from build123d import *

# Parameters (mm, degrees)
SKETCH_1_W                         = 321
SKETCH_1_H                         = 60
SM_BASE_FLANGE_1_DEPTH             = 1.5
SM_EDGE_FLANGE_1_STRIP_W           = 6.2
SM_EDGE_FLANGE_1_STRIP_H           = 1.5
SM_EDGE_FLANGE_1_STRIP_CUT_DEPTH   = 321
SM_EDGE_FLANGE_1_STRIP_2_W         = 6.2
SM_EDGE_FLANGE_1_STRIP_2_H         = 1.5
SM_EDGE_FLANGE_1_STRIP_CUT_2_DEPTH = 321
SM_EDGE_FLANGE_1_DEPTH             = 321
SM_EDGE_FLANGE_1_BEND_DEPTH        = 321
SM_EDGE_FLANGE_2_STRIP_W           = 6.2
SM_EDGE_FLANGE_2_STRIP_H           = 1.5
SM_EDGE_FLANGE_2_STRIP_CUT_DEPTH   = 321
SM_EDGE_FLANGE_2_STRIP_2_W         = 6.2
SM_EDGE_FLANGE_2_STRIP_2_H         = 1.5
SM_EDGE_FLANGE_2_STRIP_CUT_2_DEPTH = 321
SM_EDGE_FLANGE_2_DEPTH             = 321
SM_EDGE_FLANGE_2_BEND_DEPTH        = 321
CUT_EXTRUDE_2_DEPTH                = 174.385408844
CUT_EXTRUDE_3_DEPTH                = 57
CUT_EXTRUDE_3_DEPTH_BACK           = 10
SKETCH_20_W                        = 341.087454661
SKETCH_20_H                        = 74.910603127
CUT_EXTRUDE_4_DEPTH                = 166.663061664
CUT_EXTRUDE_4_DEPTH_BACK           = 166.663061664
SKETCH_21_R                        = 0.75


# Sheet-metal steps are written as plain solids
with BuildPart() as part:
    # Sketch 1 → 基体-法兰1 (new body)
    with BuildSketch(Plane.XY):
        Rectangle(SKETCH_1_W, SKETCH_1_H)
    extrude(amount=-SM_BASE_FLANGE_1_DEPTH)

    # 边线-法兰1 strip (across the edge) → 边线-法兰1 strip cut (cut)
    with BuildSketch(Plane(origin=(160.5, 30, 0), x_dir=(0, -1, 0), z_dir=(-1, 0, 0))):
        with Locations((-1.5, -0.75)):
            Rectangle(SM_EDGE_FLANGE_1_STRIP_W, SM_EDGE_FLANGE_1_STRIP_H)
    extrude(amount=SM_EDGE_FLANGE_1_STRIP_CUT_DEPTH, mode=Mode.SUBTRACT)

    # 边线-法兰1 strip 2 (across the edge) → 边线-法兰1 strip cut 2 (cut)
    with BuildSketch(Plane(origin=(-160.5, -30, 0), x_dir=(0, 1, 0), z_dir=(1, 0, 0))):
        with Locations((-1.5, -0.75)):
            Rectangle(SM_EDGE_FLANGE_1_STRIP_2_W, SM_EDGE_FLANGE_1_STRIP_2_H)
    extrude(amount=SM_EDGE_FLANGE_1_STRIP_CUT_2_DEPTH, mode=Mode.SUBTRACT)

    # 边线-法兰1 section (across the edge) → 边线-法兰1 (add)
    with BuildSketch(Plane(origin=(160.5, 30, 0), x_dir=(0, -1, 0), z_dir=(-1, 0, 0))):
        with BuildLine():
            Line((0, 0.1), (0, 26.5))
            Line((0, 26.5), (1.5, 26.5))
            Line((1.5, 26.5), (1.5, 0.1))
            ThreePointArc((1.5, 0.1), (1.529289322, 0.029289322), (1.6, 0))
            Line((1.6, 0), (1.6, -1.5))
            ThreePointArc((1.6, -1.5), (0.46862915, -1.03137085), (0, 0.1))
        make_face()
    extrude(amount=SM_EDGE_FLANGE_1_DEPTH)

    # 边线-法兰1 section 2 (across the edge) → 边线-法兰1 bend (add)
    with BuildSketch(Plane(origin=(-160.5, -30, 0), x_dir=(0, 1, 0), z_dir=(1, 0, 0))):
        with BuildLine():
            Line((0, 0.1), (0, 26.5))
            Line((0, 26.5), (1.5, 26.5))
            Line((1.5, 26.5), (1.5, 0.1))
            ThreePointArc((1.5, 0.1), (1.529289322, 0.029289322), (1.6, 0))
            Line((1.6, 0), (1.6, -1.5))
            ThreePointArc((1.6, -1.5), (0.46862915, -1.03137085), (0, 0.1))
        make_face()
    extrude(amount=SM_EDGE_FLANGE_1_BEND_DEPTH)

    # 边线-法兰2 strip (across the edge) → 边线-法兰2 strip cut (cut)
    with BuildSketch(Plane(origin=(160.5, 28.5, 26.5), x_dir=(0, 0, -1), z_dir=(-1, 0, 0))):
        with Locations((-1.5, -0.75)):
            Rectangle(SM_EDGE_FLANGE_2_STRIP_W, SM_EDGE_FLANGE_2_STRIP_H)
    extrude(amount=SM_EDGE_FLANGE_2_STRIP_CUT_DEPTH, mode=Mode.SUBTRACT)

    # 边线-法兰2 strip 2 (across the edge) → 边线-法兰2 strip cut 2 (cut)
    with BuildSketch(Plane(origin=(-160.5, -28.5, 26.5), x_dir=(0, 0, -1), z_dir=(1, 0, 0))):
        with Locations((-1.5, -0.75)):
            Rectangle(SM_EDGE_FLANGE_2_STRIP_2_W, SM_EDGE_FLANGE_2_STRIP_2_H)
    extrude(amount=SM_EDGE_FLANGE_2_STRIP_CUT_2_DEPTH, mode=Mode.SUBTRACT)

    # 边线-法兰2 section (across the edge) → 边线-法兰2 (add)
    with BuildSketch(Plane(origin=(160.5, 28.5, 26.5), x_dir=(0, 0, -1), z_dir=(-1, 0, 0))):
        with BuildLine():
            Line((0, 0.1), (0, 8.5))
            Line((0, 8.5), (1.5, 8.5))
            Line((1.5, 8.5), (1.5, 0.1))
            ThreePointArc((1.5, 0.1), (1.529289322, 0.029289322), (1.6, 0))
            Line((1.6, 0), (1.6, -1.5))
            ThreePointArc((1.6, -1.5), (0.46862915, -1.03137085), (0, 0.1))
        make_face()
    extrude(amount=SM_EDGE_FLANGE_2_DEPTH)

    # 边线-法兰2 section 2 (across the edge) → 边线-法兰2 bend (add)
    with BuildSketch(Plane(origin=(-160.5, -28.5, 26.5), x_dir=(0, 0, -1), z_dir=(1, 0, 0))):
        with BuildLine():
            Line((0, 0.1), (0, 8.5))
            Line((0, 8.5), (1.5, 8.5))
            Line((1.5, 8.5), (1.5, 0.1))
            ThreePointArc((1.5, 0.1), (1.529289322, 0.029289322), (1.6, 0))
            Line((1.6, 0), (1.6, -1.5))
            ThreePointArc((1.6, -1.5), (0.46862915, -1.03137085), (0, 0.1))
        make_face()
    extrude(amount=SM_EDGE_FLANGE_2_BEND_DEPTH)

    # 草图19 → 切除-拉伸2 (cut, through all)
    with BuildSketch(Plane(origin=(0, 30, 0), x_dir=(1, 0, 0), z_dir=(0, 1, 0))):
        with BuildLine():
            Line((-132, -5), (-18, -5))
            ThreePointArc((-18, -5), (-15.878679656, -5.878679656), (-15, -8))
            Line((-15, -8), (-15, -17))
            ThreePointArc((-15, -17), (-15.878679656, -19.121320344), (-18, -20))
            Line((-18, -20), (-132, -20))
            ThreePointArc((-132, -20), (-134.121320344, -19.121320344), (-135, -17))
            Line((-135, -17), (-135, -8))
            ThreePointArc((-135, -8), (-134.121320344, -5.878679656), (-132, -5))
        make_face()
    cut_extrude_2 = extrude(amount=-CUT_EXTRUDE_2_DEPTH, mode=Mode.SUBTRACT)

    # 镜向1: 切除-拉伸2 across plane
    add(cut_extrude_2.mirror(Plane(origin=(0, 0, 0), x_dir=(0, 0, 1), z_dir=(1, 0, 0))), mode=Mode.SUBTRACT)

    # 草图20 → 切除-拉伸3 (cut, two sides: drawn at the far end of the back side and taken through both)
    with BuildSketch(Plane.XY.offset(-CUT_EXTRUDE_3_DEPTH_BACK)):
        with Locations((-10.043727331, -17.455301564)):
            Rectangle(SKETCH_20_W, SKETCH_20_H)
    extrude(amount=CUT_EXTRUDE_3_DEPTH + CUT_EXTRUDE_3_DEPTH_BACK, mode=Mode.SUBTRACT)

    # 草图21 → 切除-拉伸4 (cut, two sides: drawn at the far end of the back side and taken through both)
    with BuildSketch(Plane.XY.offset(26.5).offset(-CUT_EXTRUDE_4_DEPTH_BACK)):
        with Locations(Location((75, 23, 0), (0, 0, 270))):
            Circle(SKETCH_21_R)
        with Locations(Location((-75, 23, 0), (0, 0, 270))):
            Circle(SKETCH_21_R)
    extrude(amount=CUT_EXTRUDE_4_DEPTH + CUT_EXTRUDE_4_DEPTH_BACK, mode=Mode.SUBTRACT)


solid = part.part
Check sheet for the modelled part. Datum: model origin and axes. Units: mm. A direction names the side the tool comes from. Give positions to 0.01 mm unless a question says otherwise; leave off trailing zeros. Write each loop counter-clockwise with the first axis right and the second up, starting at its lowest first coordinate (ties: lowest second). Pieces come first, ordered by that corner, then holes. Notation, with made-up numbers: (-21.5, 23.25) -> (31.5, 23.25) arc R21 cw to (31.5, 46.25) -> close; hole circle Ø5 at (-37, -2). An arc over 180 degrees is marked (long way). Use one line per item in the form item = value. Start each with the question number.
1. Mould release check, pull along Z, two halves, no side actions. Record for faces 3 (the flat face through (-2, 24, -1.5)), 4 (the flat face through (-2, 24, 0)), 5 (the flat face through (2, 24, 26.5)), 6 (the flat face through (160.5, 29, 10)): pulls with the +Z half, pulls with the -Z half, needs draft (parallel to the pull), parting line crosses it, or undercut.
2. Section check A-A (y = 25.5). Record the cut outline in (x, z).
3. Access from +Z, -Z, +X, -X, +Y, -Y to the whole of each face (thin tool, end or side, straight path). Record for faces 1 (the flat face through (2, 28.5, 13)), 2 (the flat face through (2, 30, 12)).
4. Thickness scan on line 1 along X through (y, z) = (23, 25.5); line 2 along Z through (x, y) = (-4.5, 23.5); line 3 along Y through (x, z) = (75, -0.25). Record the ranges inside material, lowest first. Write a range as from..to.
5. Go/stop test with flat-tipped pins: P1, Ø1.7, axis at x = 75, y = 23, coming from the -Z side; P2, Ø0.8, axis at x = 98, y = 29, coming from the +Z side. Record where each tip stops, or that it passes through.
6. Section check B-B (x = -28.5). Record the cut outline in (y, z), and give its area (3 significant figures).
Conclusion:
q1.face_3 = pulls with the -Z half
q1.face_4 = undercut
q1.face_5 = pulls with the +Z half
q1.face_6 = needs draft
q2.outline = (-160.5, -1.5) -> (160.5, -1.5) -> (160.5, 0) -> (-160.5, 0) -> close; (-160.5, 25) -> (160.5, 25) -> (160.5, 26.5) -> (-160.5, 26.5) -> close
q3.face_1 = +X, -X, -Y
q3.face_2 = +Z, -Z, +X, -X, +Y
q4.line_1 = -160.5..-75.75, -74.25..74.25, 75.75..160.5
q4.line_2 = -1.5..0, 25..26.5
q4.line_3 = 20..22.25, 23.75..29.96
q5.P1 = -1.5
q5.P2 = 26.49
q6.outline = (20, -1.5) -> (28.4, -1.5) arc R1.6 ccw to (30, 0.1) -> (30, 5) -> (28.5, 5) -> (28.5, 0.1) arc R0.1 cw to (28.4, 0) -> (20, 0) -> close; (20, 25) -> (28.4, 25) arc R0.1 cw to (28.5, 24.9) -> (28.5, 20) -> (30, 20) -> (30, 24.9) arc R1.6 ccw to (28.4, 26.5) -> (20, 26.5) -> close
q6.area = 43.9 mm²
